Part model, mm, in its own coordinate system. A direction names the side the tool comes from. Give positions to 0.01 mm unless a question says otherwise; leave off trailing zeros. Order: outer loops, then holes, each group sorted by start corner. A loop starts at its lowest first (then second) coordinate and runs counter-clockwise, first axis right, second up. Notation, with made-up numbers: M 55.25,-14 L 113.25,-14 A7 ccw 113.25,-9 Z; hole C -4,-38 d6. An arc over 180 degrees is marked long. Answer as a JSON object with one key per item and string values.
from build123d import *

# Parameters (mm, degrees)
F1_DEPTH = 40.56158
F2_DEPTH = 5.38948
F0_W     = 12.0462047143
F0_H     = 8.1998697145
F3_DEPTH = 9.06237


with BuildPart() as f1:
    # F0 (on Front) → F1 (new body, symmetric)
    with BuildSketch(Plane.XZ):
        Polygon((-14.8684419692, -13.1286175627), (-56.6685722546, -13.1286175627), (-56.6685722546, -29.630266222), (-6.6685722546, -29.630266222), (-6.6685722546, -13.1286175627), align=None)
    extrude(amount=F1_DEPTH, both=True)

    # F0 (on Front) → F2 (join, symmetric)
    with BuildSketch(Plane.XZ):
        with BuildLine():
            add(Edge.make_bspline(
                [(-56.6685722546, -13.1286175627), (-54.7797419131, 6.6462885588), (-22.0853742212, 20.4196609557), (4.3314277454, 20.0712521518)],
                knots=[0, 0, 0, 0, 69.4494877523, 69.4494877523, 69.4494877523, 69.4494877523], degree=3))
            Line((-56.6685722546, -13.1286175627), (-14.8684419692, -13.1286175627))
            Line((-14.8684419692, -13.1286175627), (-14.8684419692, 0.8713824373))
            ThreePointArc((-14.8684419692, 0.8713824373), (-9.2449303277, 14.4477405103), (4.3314277454, 20.0712521518))
        make_face()
    extrude(amount=F2_DEPTH, both=True)

    # F0 (on Front) → F3 (join, symmetric)
    with BuildSketch(Plane.XZ):
        with BuildLine():
            Line((-14.8684419692, 0.8713824373), (-14.8684419692, -13.1286175627))
            Line((-14.8684419692, -13.1286175627), (-6.6685722546, -13.1286175627))
            Line((-6.6685722546, -13.1286175627), (-6.6685722546, 0.8713824373))
            ThreePointArc((-6.6685722546, 0.8713824373), (-3.4467468477, 8.6495570304), (4.3314277454, 11.8713824373))
            Line((4.3314277454, 11.8713824373), (4.3880510932, 11.8713824373))
            Line((4.3880510932, 11.8713824373), (4.3880510932, 20.0712521518))
            Line((4.3880510932, 20.0712521518), (4.3314277454, 20.0712521518))
            ThreePointArc((4.3314277454, 20.0712521518), (-9.2449303277, 14.4477405103), (-14.8684419692, 0.8713824373))
        make_face()
        with Locations((10.4111534504, 15.9713172946)):
            Rectangle(F0_W, F0_H)
    extrude(amount=F3_DEPTH, both=True)


solid = f1.part
1. Cut at A-A on y = 22. Give the cut face in (x, z).
Worked answers:
{"outline": "M -56.67,-29.63 L -6.67,-29.63 L -6.67,-13.13 L -56.67,-13.13 Z"}
2. Probe line 1 along Y through (x, z) = (9.5, 14); line 2 along Z through (x, y) = (-39, -35.5); line 3 along Y through (x, z) = (-33.5, -12.5). List the from-to ranges inside material, lowest first.
Worked answers:
{"line 1": "y = -9.06 to 9.06", "line 2": "z = -29.63 to -13.13", "line 3": "y = -5.39 to 5.39"}
3. Which spindle directions (+Z, -Z, +X, -X, +Y, -Y) get a long thin tool onto all of the face, cutting with end or side? Do faces 1 (the flat face through (-6, 9.062, 7)), 2 (the flat face through (-33, -5.389, 0)), 3 (the flat face through (-6.669, -1, -18)). Say none if no direction does.
Worked answers:
{"face 1": "+Z, +X, -X, +Y", "face 2": "+Z, -X, -Y", "face 3": "-Z, +X, +Y, -Y"}
4. Pin check, flat tips, straight feed: P1, Ø1.1, axis at y = 8, z = -8, coming from the -X side; P2, Ø9, axis at y = 16.5, z = -9, coming from the +X side; P3, Ø6, axis at x = 8.5, y = 2.5, coming from the -Z side. Stop position of each tip, or through.
Worked answers:
{"P1": "stops at x = -14.87", "P2": "stops at x = -6.67", "P3": "stops at z = 11.87"}
5. Cut at B-B on z = -22. Give the cut face in (x, y).
Worked answers:
{"outline": "M -56.67,-40.56 L -6.67,-40.56 L -6.67,40.56 L -56.67,40.56 Z"}
